```python
from build123d import *

# Parameters (mm, degrees)
BOSS_EXTRUDE1_DEPTH = 16.51
SKETCH2_R           = 22.225
CUT_EXTRUDE1_DEPTH  = 17.51
SKETCH4_OUTSIDE_W   = 78.892
SKETCH4_OUTSIDE_H   = 78.892
SKETCH4_OUTSIDE_R   = 24.765
CUT_EXTRUDE2_DEPTH  = 6.35
CUT_EXTRUDE3_DEPTH  = 7.62
CIRPATTERN1_COUNT   = 4


with BuildPart() as part:
    # Sketch1 → Boss-Extrude1 (new body)
    with BuildSketch(Plane.XY):
        with BuildLine():
            Line((-27.305, 29.845), (27.305, 29.845))
            ThreePointArc((27.305, 29.845), (29.101051224, 29.101051224), (29.845, 27.305))
            Line((29.845, 27.305), (29.845, -27.305))
            ThreePointArc((29.845, -27.305), (29.101051224, -29.101051224), (27.305, -29.845))
            Line((27.305, -29.845), (-27.305, -29.845))
            ThreePointArc((-27.305, -29.845), (-29.101051224, -29.101051224), (-29.845, -27.305))
            Line((-29.845, -27.305), (-29.845, 27.305))
            ThreePointArc((-29.845, 27.305), (-29.101051224, 29.101051224), (-27.305, 29.845))
        make_face()
    extrude(amount=BOSS_EXTRUDE1_DEPTH)

    # Sketch2 → Cut-Extrude1 (cut, through all)
    with BuildSketch(Plane.XY.offset(16.51)):
        Circle(SKETCH2_R)
    extrude(amount=-CUT_EXTRUDE1_DEPTH, mode=Mode.SUBTRACT)

    # Sketch4 outside → Cut-Extrude2 (cut)
    with BuildSketch(Plane(origin=(0, 0, 0), x_dir=(-1, 0, 0), z_dir=(0, 0, -1))):
        Rectangle(SKETCH4_OUTSIDE_W, SKETCH4_OUTSIDE_H)
        Circle(SKETCH4_OUTSIDE_R, mode=Mode.SUBTRACT)
    extrude(amount=-CUT_EXTRUDE2_DEPTH, mode=Mode.SUBTRACT)

    # Sketch3 → Cut-Extrude3 (cut)
    with BuildSketch(Plane.XY.offset(16.51)):
        with BuildLine():
            Line((24.765, -27.305), (-24.765, -27.305))
            ThreePointArc((-24.765, -27.305), (-26.561051224, -26.561051224), (-27.305, -24.765))
            Line((-27.305, -24.765), (-27.305, 24.765))
            ThreePointArc((-27.305, 24.765), (-26.561051224, 26.561051224), (-24.765, 27.305))
            Line((-24.765, 27.305), (24.765, 27.305))
            ThreePointArc((24.765, 27.305), (26.561051224, 26.561051224), (27.305, 24.765))
            Line((27.305, 24.765), (27.305, -24.765))
            ThreePointArc((27.305, -24.765), (26.561051224, -26.561051224), (24.765, -27.305))
        make_face()
    extrude(amount=-CUT_EXTRUDE3_DEPTH, mode=Mode.SUBTRACT)

    # Sketch6 → #4 Clearance Hole1 (revolve, cut)
    with BuildSketch(Plane(origin=(-23.348665915, 23.348665915, 8.89), x_dir=(0, -1, 0), z_dir=(1, 0, 0))):
        Polygon((0, 0), (0, 8.575174487), (1.63195, 7.5946), (1.63195, 0), align=None)
    f_4_clearance_hole1 = revolve(axis=Axis((-23.348665915, 23.348665915, 15.24), (0, 0, -1)), mode=Mode.SUBTRACT)

    # CirPattern1: #4 Clearance Hole1 ×4 about axis
    cirpattern1_axis = Axis((0, 0, 0), (0, 0, 1))
    for i in range(1, CIRPATTERN1_COUNT):
        add(f_4_clearance_hole1.rotate(cirpattern1_axis, i * 360 / CIRPATTERN1_COUNT), mode=Mode.SUBTRACT)


solid = part.part
```
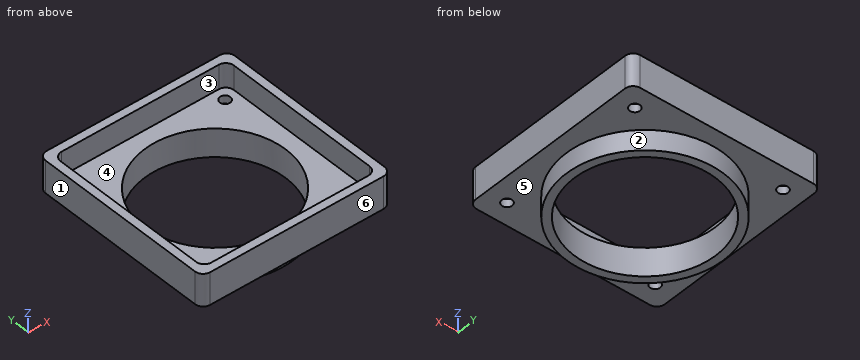
For this review, take the finished solid that the model builds, in its own axes (mm). Face numbers are marked on the shaded views. A direction names the side the tool comes from. Coordinates: 2 decimals unless noted, no trailing zeros. Loops run counter-clockwise (first coordinate to the right, second up) from the corner with the lowest first, then second, coordinate; pieces in that order, holes last. Notation, with made-up numbers: (46, 7.25) - (60, 7.25) arc R13 cw to (60, 29.25) - close; hole circle Ø1 at (81.25, 68). An arc over 180 degrees is marked (long way). Use one line per item in the form item = value. Start each with the question number.
1) Draft analysis for pull direction Y (two halves, no side actions). For the marked faces 4, 5 and 6, state which applies: released by +Y, released by -Y, zero draft, split by the parting line, or undercut.
2) To check wall thickness, follow probe 1 along X at (y, z) = (17.5, 13.5) (3 decimals); probe 2 along X at (y, z) = (-23, 7) (3 decimals). State the ranges of each line that lie inside material, in increasing order. Write a range as from..to.
3) For the marked faces 1, 2 and 3, list the 3-axis set-ups (+Z, -Z, +X, -X, +Y, -Y) from which the entire face can be reached by the end or side of a thin tool; tool diameter is ignored.
4) For pin 1 (4 mm diameter, centred on x = -23.35, y = -23.35, fed in from -Z); pin 2 (4 mm diameter, centred on y = 10.5, z = 4, fed in from -X), all flat-tipped, find the tip position at first contact; note any pin that passes through.
5) Take a section at C-C (z = 13.25). State the section outline as (x, y) points (3 decimals), plus the area to 3 significant figures.
6) Take a section at D-D (z = 3.75). State the section outline as (x, y) points (3 decimals).
7) Take a section at A-A (x = 0). State the section outline as (y, z) points (3 decimals).
From the geometry:
q1.face_4 = undercut
q1.face_5 = zero draft
q1.face_6 = released by -Y
q2.probe_1 = -29.845..-27.305, 27.305..29.845
q2.probe_2 = -29.845..-24.943, -21.754..21.754, 24.943..29.845
q3.face_1 = +Z, -Z, -X, +Y, -Y
q3.face_2 = -Z
q3.face_3 = +Z
q4.pin_1 = 6.35
q4.pin_2 = -23.26
q5.outline = (-29.845, -27.305) arc R2.54 ccw to (-27.305, -29.845) - (27.305, -29.845) arc R2.54 ccw to (29.845, -27.305) - (29.845, 27.305) arc R2.54 ccw to (27.305, 29.845) - (-27.305, 29.845) arc R2.54 ccw to (-29.845, 27.305) - close; hole (-27.305, -24.765) arc R2.54 ccw to (-24.765, -27.305) - (24.765, -27.305) arc R2.54 ccw to (27.305, -24.765) - (27.305, 24.765) arc R2.54 ccw to (24.765, 27.305) - (-24.765, 27.305) arc R2.54 ccw to (-27.305, 24.765) - close
q5.area = 581 mm2
q6.outline = circle Ø49.53 at (0, 0); hole circle Ø44.45 at (0, 0)
q7.outline = (-29.845, 6.35) - (-24.765, 6.35) - (-24.765, 0) - (-22.225, 0) - (-22.225, 8.89) - (-27.305, 8.89) - (-27.305, 16.51) - (-29.845, 16.51) - close; (22.225, 0) - (24.765, 0) - (24.765, 6.35) - (29.845, 6.35) - (29.845, 16.51) - (27.305, 16.51) - (27.305, 8.89) - (22.225, 8.89) - close
